Part model, mm, in its own coordinate system. A direction names the side the tool comes from. Give positions to 0.01 mm unless a question says otherwise; leave off trailing zeros. Order: outer loops, then holes, each group sorted by start corner. A loop starts at its lowest first (then second) coordinate and runs counter-clockwise, first axis right, second up. Notation, with made-up numbers: (80.25, 34.5) - (84.25, 34.5) arc R23 cw to (84.25, 47.5) - close; hole circle Ø2 at (39, 28). An arc over 180 degrees is marked (long way). One line per item, written item: value.
```python
from build123d import *

# Parameters (mm, degrees)
F0_W     = 80.713644
F0_H     = 152.196348
F1_DEPTH = 12.7
F2_R     = 5
F3_T     = -2.54


with BuildPart() as f1:
    # F0 (on Front) → F1 (new body, symmetric)
    with BuildSketch(Plane.XZ):
        Rectangle(F0_W, F0_H)
    extrude(amount=F1_DEPTH, both=True)

    # F2
    f2_edges = [f1.edges().sort_by_distance(p)[0] for p in [
        (-40.356822, 0, 76.098174),
        (40.356822, 0, 76.098174),
        (40.356822, 0, -76.098174),
        (-40.356822, 0, -76.098174),
    ]]
    fillet(f2_edges, radius=F2_R)

    # F3
    f3_openings = [f1.faces().sort_by_distance(p)[0] for p in [
        (0, -12.7, 0),
    ]]
    offset(amount=F3_T, openings=f3_openings)


solid = f1.part
```
1) Mould opens along X. For faces 3 (the cylindrical face through (38.931, 0.178, 74.595)), 4 (the flat face through (-39, -12.7, 23)), 5 (the flat face through (-37.817, -1, -1)), 6 (the flat face through (-40.357, 0, -1)) say: released by +X, released by -X, zero draft, split by the parting line, or undercut.
Outcome:
face 3: released by +X
face 4: zero draft
face 5: undercut
face 6: released by -X
2) Cut at A-A, the plane y = -8. Give the cut face in (x, z), then the cut area to 3 significant figures.
Outcome:
outline: (-40.36, -71.1) arc R5 ccw to (-35.36, -76.1) - (35.36, -76.1) arc R5 ccw to (40.36, -71.1) - (40.36, 71.1) arc R5 ccw to (35.36, 76.1) - (-35.36, 76.1) arc R5 ccw to (-40.36, 71.1) - close; hole (-37.82, -71.1) arc R2.46 ccw to (-35.36, -73.56) - (35.36, -73.56) arc R2.46 ccw to (37.82, -71.1) - (37.82, 71.1) arc R2.46 ccw to (35.36, 73.56) - (-35.36, 73.56) arc R2.46 ccw to (-37.82, 71.1) - close
area: 1,140 mm^2
3) Cut at B-B, the plane x = -27. Give the cut face in (y, z).
Outcome:
outline: (-12.7, -76.1) - (12.7, -76.1) - (12.7, 76.1) - (-12.7, 76.1) - (-12.7, 73.56) - (10.16, 73.56) - (10.16, -73.56) - (-12.7, -73.56) - close
4) Cut at C-C, the plane z = 16. Give the cut face in (x, y).
Outcome:
outline: (-40.36, -12.7) - (-37.82, -12.7) - (-37.82, 10.16) - (37.82, 10.16) - (37.82, -12.7) - (40.36, -12.7) - (40.36, 12.7) - (-40.36, 12.7) - close
5) Which spindle directions (+Z, -Z, +X, -X, +Y, -Y) get a long thin tool onto all of the face, cutting with end or side? Do faces 1 (the flat face through (0, -1, -73.558)), 2 (the cylindrical face through (38.931, -0.178, -74.595)). Say none if no direction does.
Outcome:
face 1: -Y
face 2: -Z, +X, +Y, -Y
6) Drill centre lines: line 1 along X through (y, z) = (-11, -69); line 2 along Z through (x, y) = (22, -11.25); line 3 along Y through (x, z) = (21, -9). Where is each one in solid material? Low to high. Write a range as from..to.
Outcome:
line 1: x = -40.36..-37.82, 37.82..40.36
line 2: z = -76.1..-73.56, 73.56..76.1
line 3: y = 10.16..12.7
7) Pin check, flat tip, straight feed: pin 1 (6 mm diameter, centred on x = 16.5, z = 12, fed in from -Y). Stop position of the tip, or through.
Outcome:
pin 1: stops at y = 10.16
